from build123d import *

# Parameters (mm, degrees)
SKETCH019_R     = 19
SKETCH019_R_2   = 17
PAD009003_DEPTH = 7
SKETCH017_R     = 28
SKETCH017_R_2   = 19
PAD009004_DEPTH = 2
SKETCH018_R     = 2
PAD009005_DEPTH = 7
SKETCH020_R     = 2
POCKET003_DEPTH = 5


with BuildPart() as part:
    # Sketch019 → Pad009003 (new body)
    with BuildSketch(Plane.XY):
        Circle(SKETCH019_R)
        Circle(SKETCH019_R_2, mode=Mode.SUBTRACT)
    extrude(amount=PAD009003_DEPTH)

    # Sketch017 → Pad009004 (join)
    with BuildSketch(Plane(origin=(0, 0, 0), x_dir=(1, 0, 0), z_dir=(0, 0, -1))):
        Circle(SKETCH017_R)
        Circle(SKETCH017_R_2, mode=Mode.SUBTRACT)
    extrude(amount=-PAD009004_DEPTH)

    # Sketch018 → Pad009005 (join)
    with BuildSketch(Plane.XY):
        with Locations((22.25, 0)):
            Circle(SKETCH018_R)
        with Locations((-11.125, 19.269065)):
            Circle(SKETCH018_R)
        with Locations((-11.125, -19.269065)):
            Circle(SKETCH018_R)
    extrude(amount=PAD009005_DEPTH)

    # Sketch020 → Pocket003 (cut)
    with BuildSketch(Plane.XY.offset(2.2)):
        with Locations((-22.25, 0)):
            Circle(SKETCH020_R)
    extrude(amount=-POCKET003_DEPTH, mode=Mode.SUBTRACT)


solid = part.part
The listing builds one solid part. Answer for the finished solid, in the listing's coordinates (mm). A direction names the side the tool comes from. Round coordinates to 2 decimals unless told otherwise and drop trailing zeros. Loops run counter-clockwise (first coordinate to the right, second up) from the corner with the lowest first, then second, coordinate; pieces in that order, holes last. Notation, with made-up numbers: M -3.5,-13.75 L 44.5,-13.75 A21 cw 44.5,-8.75 Z; hole C 28.25,83.25 d9. An arc over 180 degrees is marked long. Write each question's results on one line, items separated by ' | '. Start each with the question number.
1) Determine the mould class of faces 1 (the flat face through (22, 0, 7)), 2 (the cylindrical face through (-12.71, 18.05, 4.46)), 3 (the cylindrical face through (25.865, 10.724, 0.986)) for opening direction X: pulls with the +X half, pulls with the -X half, needs draft (parallel to the pull), parting line crosses it, or undercut.
2) Which of the six approach directions +Z, -Z, +X, -X, +Y, -Y give full straight-line access (tool end or side, diameter ignored) to faces 4 (the cylindrical face through (9.139, 14.334, 3.451)), 5 (the cylindrical face through (8.767, -16.856, 4.465))?
3) Find section C-C on z = 5. Write down the section's boundary in (x, y) (3 decimals), plus the area to 3 significant figures.
4) Straight lines are drawn through the part: probe 1 along Y at (x, z) = (-22.25, 1.5); probe 2 along X at (y, z) = (-1, 1.5); probe 3 along Y at (x, z) = (0, 4.5). For each, find the intervals that lie inside material, in ascending order.
5) Find section A-A on y = 0. Write down the section's boundary in (x, z), plus the area to 3 significant figures.
6) Find section B-B on x = 0. Write down the section's boundary in (y, z), plus the area to 3 significant figures.
7) Each of these flat-tipped pins is pushed along its axis until it touches: pin 1 (3 mm diameter, centred on x = -15, z = 3, fed in from -Y); pin 2 (10 mm diameter, centred on x = 1, y = 19.5, fed in from -Z); pin 3 (1.5 mm diameter, centred on y = 14.5, z = 5, fed in from +X); pin 4 (3 mm diameter, centred on x = -22.25, y = 0, fed in from +Z). Where does it stop, or does it pass through?
8) Find section D-D on z = 1. Write down the section's boundary in (x, y).
Final values:
1) face 1: needs draft | face 2: undercut | face 3: parting line crosses it
2) face 4: +Z, -Z | face 5: +Z
3) outline: C 0,0 d38; C -11.125,-19.269 d4; C -11.125,19.269 d4; C 22.25,0 d4; hole C 0,0 d34 | area: 264 mm²
4) probe 1: -17 to -2, 2 to 17 | probe 2: -27.98 to -23.98, -20.52 to -16.97, 16.97 to 27.98 | probe 3: -19 to -17, 17 to 19
5) outline: M -28,0 L -24.25,0 L -24.25,2 L -28,2 Z; M -20.25,0 L -17,0 L -17,7 L -19,7 L -19,2 L -20.25,2 Z; M 17,0 L 28,0 L 28,2 L 24.25,2 L 24.25,7 L 20.25,7 L 20.25,2 L 19,2 L 19,7 L 17,7 Z | area: 76.0 mm²
6) outline: M -28,0 L -17,0 L -17,7 L -19,7 L -19,2 L -28,2 Z; M 17,0 L 28,0 L 28,2 L 19,2 L 19,7 L 17,7 Z | area: 64.0 mm²
7) pin 1: y = -24.32 | pin 2: z = 0 | pin 3: x = 13.11 | pin 4: through
8) outline: C 0,0 d56; hole C -22.25,0 d4; hole C 0,0 d34
